from build123d import *

# Parameters (mm, degrees)
F0_W     = 5.8
F0_H     = 2
F1_DEPTH = 20
F2_R     = 10
F3_SIZE  = 0.49999


# Not quite as in the source:
# - a fillet or chamfer is up to 0.001 mm smaller than in the source, because OpenCascade refuses the exact size


with BuildPart() as f1:
    # F0 (on Top) → F1 (new body)
    with BuildSketch(Plane.XY):
        with Locations((-39.9097009659, 46.350823313)):
            Rectangle(F0_W, F0_H)
        Polygon((-42.8097009659, 45.350823313), (-42.8097009659, 47.350823313), (-67.8097009659, 47.350823313), (-67.8097009659, 26.850823313), (-42.8097009659, 26.850823313), (-42.8097009659, 28.850823313), align=None)
        Polygon((-35.0097009659, 47.350823313), (-37.0097009659, 47.350823313), (-37.0097009659, 45.350823313), (-37.0097009659, 44.850823313), (-35.0097009659, 44.850823313), align=None)
        with Locations((-39.9097009659, 27.850823313)):
            Rectangle(F0_W, F0_H)
        Polygon((-37.0097009659, 29.350823313), (-37.0097009659, 28.850823313), (-37.0097009659, 26.850823313), (-35.0097009659, 26.850823313), (-35.0097009659, 29.350823313), align=None)
    extrude(amount=F1_DEPTH)

    # F2
    f2_edges = [f1.edges().sort_by_distance(p)[0] for p in [
        (-67.809701, 47.350823, 10),
        (-67.809701, 26.850823, 10),
    ]]
    fillet(f2_edges, radius=F2_R)

    # F3 (size 0.5 in the source; OpenCascade refuses exactly that, so slightly less here)
    f3_edges = [f1.edges().sort_by_distance(p)[0] for p in [
        (-35.009701, 47.350823, 10),
        (-35.009701, 44.850823, 10),
        (-35.009701, 29.350823, 10),
        (-35.009701, 26.850823, 10),
        (-37.009701, 29.350823, 10),
        (-37.009701, 45.350823, 10),
    ]]
    chamfer(f3_edges, length=F3_SIZE)


solid = f1.part
Geometry: final body of the model. Coordinates: model frame, mm. A direction names the side the tool comes from. Coordinates: 2 decimals unless noted, no trailing zeros. Loops run counter-clockwise (first coordinate to the right, second up) from the corner with the lowest first, then second, coordinate; pieces in that order, holes last. Notation, with made-up numbers: M 11,79.25 L 54,79.25 A17 ccw 54,103.25 Z; hole C -33,6 d6. An arc over 180 degrees is marked long. One line per item, written item: value. Start each with the question number.
1) Cut plane C-C (x = -63.5). Return loops of the section in (y, z).
2) Reachability of faces 1 (the flat face through (-36, 29.351, 10)), 2 (the flat face through (-40, 45.351, 10)), 3 (the flat face through (-52, 37, 20)) from +Z, -Z, +X, -X, +Y, -Y: full face, straight path, thin tool, end or side. Return the list, or none.
3) Cut plane B-B (y = 34.25). Return loops of the section in (x, z), then the cut area to 3 significant figures.
4) Pin query (flat end, axial travel): P1, Ø6, axis at y = 33, z = 7.5, coming from the +X side; P2, Ø10, axis at y = 44.5, z = 15, coming from the -X side; P3, Ø5, axis at y = 44, z = 14, coming from the -X side. Return the tip coordinate at first contact, or that it passes through.
5) Material intervals for L1, parallel to Y at x = -40, z = 19.25; L2, parallel to Y at x = -36.5, z = 10.5; L3, parallel to Y at x = -58, z = 12.25, sorted ascending. Write a range as from..to.
6) Draft query along Y for faces 4 (the cylindrical face through (-64.8, 44.5, 10.1)), 5 (the flat face through (-36, 44.851, 10)), 6 (the flat face through (-35.01, 28, 10)). Return one class per face: released by +Y, released by -Y, zero draft, split by the parting line, or undercut.
Evaluation:
1. outline: M 28.63,0 L 45.57,0 L 45.57,20 L 28.63,20 Z
2. face 1: +Z, -Z, +X
2. face 2: +Z, -Z
2. face 3: +Z, +X, -X, +Y, -Y
3. outline: M -67.47,0 L -42.81,0 L -42.81,20 L -67.47,20 Z
3. area: 493 mm^2
4. P1: x = -42.81
4. P2: x = -67.58
4. P3: x = -66.91
5. L1: 26.85..28.85, 45.35..47.35
5. L2: 26.85..29.35, 44.85..47.35
5. L3: 26.85..47.35
6. face 4: released by +Y
6. face 5: undercut
6. face 6: zero draft
